from build123d import *


with BuildPart() as part:
    # Sketch1 → Revolve1 (revolve)
    with BuildSketch(Plane.XY):
        with BuildLine():
            ThreePointArc((-0.875, -1.515544457), (-0.642037087, -2.077966681), (-1.125, -2.448557159))
            Line((-1.125, -2.448557159), (-2.2, -2.448557159))
            Line((-2.2, -2.448557159), (-2.2, -3.198557159))
            Line((-2.2, -3.198557159), (-1, -3.198557159))
            Line((-1, -3.198557159), (-1, -5.698557159))
            Line((-1, -5.698557159), (0, -5.698557159))
            Line((0, -5.698557159), (0, -1.75))
            ThreePointArc((0, -1.75), (-0.452933329, -1.690370196), (-0.875, -1.515544457))
        make_face()
        with BuildLine():
            ThreePointArc((0, -1.75), (-1.75, 0), (0, 1.75))
            Line((0, 1.75), (0, -1.75))
        make_face()
    revolve(axis=Axis((0, 40.420109298, 0), (0, -1, 0)))


solid = part.part
Here's how the part is built. I have some questions about the finished solid (model axes, mm). A direction names the side the tool comes from. Coordinates: 2 decimals unless noted, no trailing zeros. Loops run counter-clockwise (first coordinate to the right, second up) from the corner with the lowest first, then second, coordinate; pieces in that order, holes last.
1. I need wall thicknesses on L1, parallel to Z at x = 0, y = -5; L2, parallel to Y at x = -0.85, z = 0.35; L3, parallel to Y at x = -1.3, z = 0.85. Which ranges of each line are inside material? Lowest first, please.
2. If we mould it in two halves opening along Y, with no side actions, what happens to faces 3 (the flat face through (0, -5.699, 0)), 4 (the cylindrical face through (0, -4, 1)), 5 (the flat face through (-1, -2.449, -1))? For each: pulls with the +Y half, pulls with the -Y half, needs draft (parallel to the pull), parting line crosses it, or undercut.
3. Imagine slicing it at A-A, the plane x = -1.45. Please give me the cut outline in (y, z).
4. Imagine slicing it at D-D, the plane y = -2.75. Please give me the cut outline in (x, z).
5. For P1, Ø1.5, axis at y = -1, z = 0, coming from the +X side; P2, Ø1.5, axis at x = -1, z = 1, coming from the +Y side, each with a flat end and sliding along its axis, tell me the tip position at first contact or that it passes through.
6. Imagine slicing it at B-B, the plane z = 1.35. Please give me the cut outline in (x, y).
7. Imagine slicing it at C-C, the plane z = 0. Please give me the cut outline in (x, y) (3 decimals).
8. For faces 1 (the cylindrical face through (-2.1, -2.83, -0.66)), 2 (the flat face through (-1, -3.199, -1)), which set-ups out of +Z, -Z, +X, -X, +Y, -Y let a thin tool reach every point of the face, with its end or its side?
Taken from the geometry:
1. L1: z = -1 to 1
1. L2: y = -5.7 to -2.4, -1.49 to 1.49
1. L3: y = -3.2 to -2.45, -0.81 to 0.81
2. face 3: pulls with the -Y half
2. face 4: needs draft
2. face 5: undercut
3. outline: (-3.2, -1.65) - (-2.45, -1.65) - (-2.45, 1.65) - (-3.2, 1.65) - close; circle Ø1.96 at (0, 0)
4. outline: circle Ø4.4 at (0, 0)
5. P1: stops at x = 1.73
5. P2: stops at y = 1.62
6. outline: (-1.74, -3.2) - (1.74, -3.2) - (1.74, -2.45) - (-1.74, -2.45) - close; circle Ø2.23 at (0, 0)
7. outline: (-2.2, -3.199) - (-1, -3.199) - (-1, -5.699) - (1, -5.699) - (1, -3.199) - (2.2, -3.199) - (2.2, -2.449) - (1.125, -2.449) arc R0.5 cw to (0.875, -1.516) arc R1.75 ccw (long way) to (-0.875, -1.516) arc R0.5 cw to (-1.125, -2.449) - (-2.2, -2.449) - close
8. face 1: +Y, -Y
8. face 2: -Y
